Check sheet for the modelled part. Datum: model origin and axes. Units: mm. A direction names the side the tool comes from. Give positions to 0.01 mm unless a question says otherwise; leave off trailing zeros. Write each loop counter-clockwise with the first axis right and the second up, starting at its lowest first coordinate (ties: lowest second). Pieces come first, ordered by that corner, then holes. Notation, with made-up numbers: (75, 20.5) - (94, 20.5) arc R20 ccw to (94, 58.5) - close; hole circle Ø10 at (2.25, -16.75). An arc over 180 degrees is marked (long way). Return JSON: item names as keys, results as strings. Group by question number.
Autodesk Inventor part; units mm, degrees
ref_plane "YZ Plane" through (0, 0, 0) normal (1, 0, 0) x (0, 1, 0)
ref_plane "XZ Plane" through (0, 0, 0) normal (0, 1, 0) x (-1, 0, 0)
ref_plane "XY Plane" through (0, 0, 0) normal (0, 0, 1) x (1, 0, 0)
sketch "スケッチ1" plane through (0, 0, 0) normal (0, 0, 1) x (1, 0, 0)
  line L0 (-50, 0) -> (50, 0) construction
  circle A0 centre (-50, 0) radius 4
  circle A1 centre (50, 0) radius 5.55
  line L1 (-50, 11.35) -> (-23, 11.35)
  line L2 (-50, -11.35) -> (50, -11.35)
  arc A2 (50, -11.35) -> (50, 11.35) centre (50, 0) ccw
  line L3 (30, 17) -> (-15, 17)
  line L4 (-15, 17) -> (-23, 11.35)
  line L5 (-24.9115, 10) -> (41.8474, 10) construction
  line L6 (-15, 17) -> (-15, 10) construction
  line L7 (30, 17) -> (30, 10) construction
  circle A3 centre (27.5, 13.5) radius 1.55
  circle A4 centre (-12.5, 13.5) radius 1.55
  circle A5 centre (7.5, 13.5) radius 1.55
  line L8 (-15, 13.5) -> (30, 13.5) construction
  line L9 (30, 16) -> (-15, 16) construction
  line L10 (-15, 16) -> (-15, 11) construction
  line L11 (-15, 11) -> (30, 11) construction
  line L12 (30, 11) -> (30, 16) construction
  line L13 (-23, 11.35) -> (50, 11.35)
  arc A6 (-50, 11.35) -> (-50, -11.35) centre (-50, 0) ccw
  line L14 (7.5, 17) -> (7.5, 10.5172) construction
  line L15 (30, 17) -> (52.8887, 10.9762)
  point P0 (0, 0)
  point P1 (0, 0)
  point P2 (55.7736, 9.7718)
  point P3 (38, 11.35)
  dimension "d0" = 100
  dimension "d1" = 8
  dimension "d8" = 11.1
  dimension "d10" = 7
  dimension "d11" = 45
  dimension "d12" = 2.5
  dimension "d13" = 3.1
  dimension "d14" = 2.5
  dimension "d15" = 20
  dimension "d17" = 5
  dimension "d18" = 11
  dimension "d69" = 11.35
  dimension "d72" = 11.35
  dimension "d87" = 8
  dimension "d88" = 8
extrude "押し出し1" add sketch "スケッチ1" along normal blind 2
fillet "フィレット1" radius 5 4 edges at (-23, 11.35, 1) (-15, 17, 1) (30, 17, 1) (-50, 11.35, 1)
sketch "スケッチ2" plane through (0, 0, 2) normal (0, 0, 1) x (1, 0, 0)
  arc A0 (50, -11.35) -> (52.8887, 10.9762) centre (50, 0) ccw
  line L0 (18, -20) -> (-35.4549, -20) construction
  line L1 (-76.9372, -11.5) -> (-72, -11.5)
  line L2 (-76.9372, -12.4) -> (-76.9372, -11.5)
  line L3 (-71.9872, -11.45) -> (-76.9872, -11.45)
  line L4 (-76.9872, -11.45) -> (-76.9872, -12.45)
  circle A1 centre (-50, 0) radius 4
  circle A2 centre (-50, 0) radius 5.5 construction
  circle A3 centre (50, 0) radius 5.55
  line L5 (83.3205, -17.7128) -> (50, 0) construction
  line L6 (50, 0) -> (18, -20) construction
  line L7 (83.3205, -17.7128) -> (37.8533, -17.7128) construction
  line L8 (-13.4166, -12.4128) -> (46.4577, -12.4128)
  line L9 (46.4577, -12.4128) -> (46.4577, -11.5128)
  line L10 (46.4577, -11.5128) -> (45.5205, -11.5128)
  line L11 (45.5205, -11.5128) -> (35.5205, -7.0128)
  line L12 (35.5205, -7.0128) -> (-2.4795, -7.0128)
  line L13 (-2.4795, -7.0128) -> (-12.4795, -11.5128)
  line L14 (-12.4795, -11.5128) -> (-13.4166, -11.5128)
  line L15 (-13.4166, -11.5128) -> (-13.4166, -12.4128)
  line L16 (-12.4902, -11.4628) -> (-2.4902, -6.9628)
  line L17 (-2.4902, -6.9628) -> (35.5312, -6.9628)
  line L18 (35.5312, -6.9628) -> (45.5312, -11.4628)
  line L19 (45.5312, -11.4628) -> (46.5077, -11.4628)
  line L20 (46.5077, -11.4628) -> (46.5077, -12.4628)
  line L21 (46.5077, -12.4628) -> (-13.4666, -12.4628)
  line L22 (-13.4666, -12.4628) -> (-13.4666, -11.4628)
  line L23 (-13.4666, -11.4628) -> (-12.4902, -11.4628)
  point P0 (56.6914, 9.1677)
  point P1 (0, 0)
  point P2 (50, 11.35)
  dimension "d19" = 20
  dimension "d20" = 32
  dimension "d32" = 11
  dimension "d33" = 120
  dimension "d37" = 37.8
  dimension "d38" = 6.2
  dimension "d39" = 0.05
  dimension "d49" = 38
  dimension "d50" = 10
  dimension "d51" = 10
  dimension "d52" = 4.5
  dimension "d53" = 0.9
  dimension "d54" = 59.9743
extrude "押し出し2" cut sketch "スケッチ2" against normal blind 10 contours L15 L14 L13 L12 L11 L10 L9 L8 | L16 L17 L18 L19 L20 L21 L22 L23
fillet "フィレット2" radius 2 4 edges at (45.2805, -11.35, 1) (-12.2395, -11.35, 1) (35.5312, -6.9628, 1) (-2.4902, -6.9628, 1)
sketch "スケッチ4" plane through (0, 0, 2) normal (0, 0, 1) x (1, 0, 0)
  circle A0 centre (50, 0) radius 5.55
  circle A1 centre (50, 0) radius 8.5 construction
  line L0 (50, 0) -> (50, 8.5) construction
  circle A2 centre (50, 8.5) radius 1.35
  circle A3 centre (41.5, 0) radius 1.35
  circle A4 centre (50, -8.5) radius 1.35
  circle A5 centre (58.5, 0) radius 1.35
  point P0 (0, 0)
  dimension "d61" = 17
  dimension "d62" = 2.7
  dimension "d65" = 360
extrude "押し出し4" cut sketch "スケッチ4" against normal through all contours A2 | A3 | A4 | A5
sketch "スケッチ6" plane through (0, 0, 2) normal (0, 0, 1) x (1, 0, 0)
  circle A0 centre (-50, 0) radius 4
  circle A1 centre (-50, 0) radius 8.5 construction
  circle A2 centre (-58.5, 0) radius 2.5
  line L0 (-50, 0) -> (-58.5, 0) construction
  line L1 (-50, 0) -> (-41.5, 0) construction
  circle A3 centre (-41.5, 0) radius 2.5
  arc A4 (-50, 11.35) -> (-50, -11.35) centre (-50, 0) ccw
  line L2 (-58.5, -2.5) -> (-61.0712, -2.5)
  line L3 (-58.5, 2.5) -> (-61.0712, 2.5)
  point P0 (0, 0)
  dimension "d78" = 17
  dimension "d79" = 5
  dimension "d82" = 360
extrude "押し出し6" cut sketch "スケッチ6" against normal through all contours A2 | A2 L2 A4 L3 | A3
fillet "フィレット4" radius 2 2 edges at (-61.0712, 2.5, 1) (-61.0712, -2.5, 1)
equation "\"d14\" = d12"
properties part number "リンク_メインフレーム_6_4" material "GFRP"
Item 1: Section check C-C on y = 8.5. Record the cut outline in (x, z).
Item 2: Section check B-B on x = -41.5. Record the cut outline in (y, z), plus the area to 3 significant figures.
Item 3: Section check A-A on y = 0. Record the cut outline in (x, z).
Item 4: Access from +Z, -Z, +X, -X, +Y, -Y to the whole of each face (thin tool, end or side, straight path). Record for faces 1 (the face through (-7.428, -9.185, 1.014)), 2 (the face through (8, 17, 1)), 3 (the face through (-37, 11.35, 1)).
Item 5: Depth check by flat-ended pin: pin 1 (1 mm diameter, centred on x = 6.5, z = 0.5, fed in from -Y); pin 2 (3.5 mm diameter, centred on x = 58.5, y = 0, fed in from -Z). Enter the tip coordinate at first touch or a pass-through.
Item 6: Material ranges on line 1 along Y through (x, z) = (7.5, 1.8); line 2 along Y through (x, z) = (-41.5, 1.4); line 3 along X through (y, z) = (-0.75, 1.25), recorded low to high. Write a range as from..to.
Item 7: Mould release check, pull along X, two halves, no side actions. Record for faces 4 (the face through (0, 3, 0)), 5 (the face through (61.283, -1.229, 0.986)), 6 (the face through (-23.09, 11.58, 1.01)), 7 (the face through (28.978, 13.034, 0.986)): +X half, -X half, draft (parallel to the pull), parting line (faces both ways), or undercut.
Item 8: Section check D-D on y = 13.5. Record the cut outline in (x, z), plus the area to 3 significant figures.
Reply:
{
 "1": {"outline": "(-57.52, 0) - (48.65, 0) - (48.65, 2) - (-57.52, 2) - close; (51.35, 0) - (57.52, 0) - (57.52, 2) - (51.35, 2) - close"},
 "2": {"outline": "(-11.35, 0) - (-2.5, 0) - (-2.5, 2) - (-11.35, 2) - close; (2.5, 0) - (11.35, 0) - (11.35, 2) - (2.5, 2) - close", "area": "35.4 mm²"},
 "3": {"outline": "(-56, 0) - (-54, 0) - (-54, 2) - (-56, 2) - close; (-46, 0) - (-44, 0) - (-44, 2) - (-46, 2) - close; (-39, 0) - (40.15, 0) - (40.15, 2) - (-39, 2) - close; (42.85, 0) - (44.45, 0) - (44.45, 2) - (42.85, 2) - close; (55.55, 0) - (57.15, 0) - (57.15, 2) - (55.55, 2) - close; (59.85, 0) - (61.35, 0) - (61.35, 2) - (59.85, 2) - close"},
 "4": {"face 1": "+Z, -Z, -Y", "face 2": "+Z, -Z, +X, -X, +Y", "face 3": "+Z, -Z, -X, +Y"},
 "5": {"pin 1": "y = -6.96", "pin 2": "z = 0"},
 "6": {"line 1": "-6.96..11.95, 15.05..17", "line 2": "-11.35..-2.5, 2.5..11.35", "line 3": "-56.12..-53.93, -46.07..-43.88, -39.12..40.38, 42.62..44.5, 55.5..57.38, 59.62..61.33"},
 "7": {"face 4": "draft", "face 5": "+X half", "face 6": "-X half", "face 7": "undercut"},
 "8": {"outline": "(-19.96, 0) - (-14.05, 0) - (-14.05, 2) - (-19.96, 2) - close; (-10.95, 0) - (5.95, 0) - (5.95, 2) - (-10.95, 2) - close; (9.05, 0) - (25.95, 0) - (25.95, 2) - (9.05, 2) - close; (29.05, 0) - (43.3, 0) - (43.3, 2) - (29.05, 2) - close", "area": "108 mm²"}
}
